For this review, take the finished solid that the model builds, in its own axes (mm). Coordinates: 2 decimals unless noted, no trailing zeros. Order: outer loops, then holes, each group sorted by start corner. A loop starts at its lowest first (then second) coordinate and runs counter-clockwise, first axis right, second up.
from build123d import *

# Parameters (mm, degrees)
SKETCH1_R           = 25.4
BOSS_EXTRUDE1_DEPTH = 127
SKETCH2_W           = 6.35
SKETCH2_H           = 6.35


with BuildPart() as part:
    # Sketch1 → Boss-Extrude1 (new body, symmetric)
    with BuildSketch(Plane.XY):
        Circle(SKETCH1_R)
    extrude(amount=BOSS_EXTRUDE1_DEPTH, both=True)

    # Sketch2 → Cut-Revolve1 (revolve, cut)
    with BuildSketch(Plane(origin=(0, 0, 0), x_dir=(0, 0, -1), z_dir=(1, 0, 0)), mode=Mode.PRIVATE) as cut_revolve1_sk:
        with Locations((0, 22.225)):
            Rectangle(SKETCH2_W, SKETCH2_H)
    revolve(cut_revolve1_sk.sketch.rotate(Axis((0, 0, 127), (0, 0, -1)), 90), axis=Axis((0, 0, 127), (0, 0, -1)), mode=Mode.SUBTRACT)  # turned: the seam where the file's is


solid = part.part
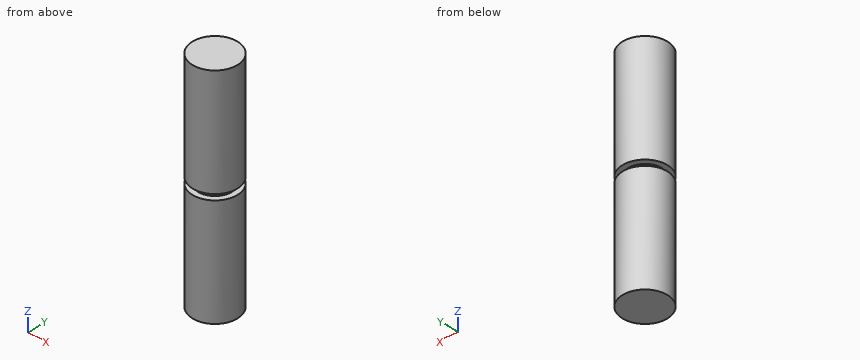
1. Clearance check with flat-ended pins moving along their axes: pin 1 Ø6 at (x, z) = (10, 11) entering from +Y; pin 2 Ø4 at (x, z) = (20, 80) entering from -Y; pin 3 Ø1.5 at (x, z) = (4, 42) entering from -Y. State where each tip first meets the part, or that it passes through.
Answer below:
pin 1: stops at y = 24.42
pin 2: stops at y = -17.92
pin 3: stops at y = -25.19
2. Take a section at C-C, the plane x = 5.5. Give the boundary of the cut face in (y, z) (3 decimals).
Answer below:
outline: (-24.797, -127) - (24.797, -127) - (24.797, -3.175) - (18.239, -3.175) - (18.239, 3.175) - (24.797, 3.175) - (24.797, 127) - (-24.797, 127) - (-24.797, 3.175) - (-18.239, 3.175) - (-18.239, -3.175) - (-24.797, -3.175) - close
3. To check wall thickness, follow L1, parallel to Z at x = -5, y = -20.5 (3 decimals); L2, parallel to Y at x = -0.5, z = 38.5; L3, parallel to X at y = 3.5, z = -111. State the ranges of each line that lie inside material, in increasing order.
Answer below:
L1: z = -127 to -3.175, 3.175 to 127
L2: y = -25.4 to 25.4
L3: x = -25.16 to 25.16
4. Take a section at B-B, the plane z = -108.5. Give the boundary of the cut face in (x, y), plus the area to 3 significant figures.
Answer below:
outline: circle Ø50.8 at (0, 0)
area: 2,030 mm2
5. Take a section at A-A, the plane y = -8. Give the boundary of the cut face in (x, z) (3 decimals).
Answer below:
outline: (-24.107, -127) - (24.107, -127) - (24.107, -3.175) - (17.289, -3.175) - (17.289, 3.175) - (24.107, 3.175) - (24.107, 127) - (-24.107, 127) - (-24.107, 3.175) - (-17.289, 3.175) - (-17.289, -3.175) - (-24.107, -3.175) - close
